Geometry: final body of the model. Coordinates: model frame, mm. A direction names the side the tool comes from. Give positions to 0.01 mm unless a question says otherwise; leave off trailing zeros. Write each loop counter-clockwise with the first axis right and the second up, starting at its lowest first coordinate (ties: lowest second). Pieces come first, ordered by that corner, then holes.
Q1. Section C-C (x = 12.5). Return the cut outline in (y, z).
Q2. Reachability of faces 4 (the cylindrical face through (-15.497, 3.441, 0.124)), 5 (the flat face through (5.474, -3.219, 3.881)), 6 (the flat face through (-10.304, 3.106, -7.638)), 7 (the cylindrical face through (-5.604, -14.23, -7.638)) from +Z, -Z, +X, -X, +Y, -Y: full face, straight path, thin tool, end or side. Return the list, or none.
Q3. Section B-B (y = -12). Return the cut outline in (x, z).
Q4. Mould query, pull axis Y, two halves, no side actions, for faces 1 (the cylindrical face through (-9.52, 11.97, -7.64)), 2 (the flat face through (7.88, -7.47, -7.64)), 3 (the flat face through (0, -13, -8.89)). Classes: +Y half, -Y half, draft (parallel to the pull), parting line (faces both ways), or undercut.
Q5. Section D-D (x = 5.5). Return the cut outline in (y, z).
Q6. Pin query (flat end, axial travel): pin 1 Ø5 at (y, z) = (4, -5.5) entering from +X; pin 2 Ø1.5 at (y, z) = (8, -5) entering from +X. Return the tip coordinate at first contact, or that it passes through.
Q7. Section A-A (z = 6). Return the cut outline in (x, y) (3 decimals).
Q8. Line query: line 1 (Y direction, x = 0, z = 2.25) (3 decimals); line 2 (X direction, y = 0, z = -0.75) (3 decimals); line 3 (Z direction, x = -4, y = -12). Output: solid intervals per line, ascending.
from build123d import *

# Parameters (mm, degrees)
BOSS_EXTRUDE1_DEPTH = 8.89
CUT_EXTRUDE1_DEPTH  = 10.16
CUT_EXTRUDE2_DEPTH  = 2.54


with BuildPart() as part:
    # Sketch1 → Boss-Extrude1 (new, symmetric)
    with BuildSketch(Plane.XY):
        with BuildLine():
            ThreePointArc((0, 15.875), (-15.875, 0), (0, -15.875))
            ThreePointArc((0, -15.875), (15.875, 0), (0, 15.875))
        make_face()
    extrude(amount=BOSS_EXTRUDE1_DEPTH, both=True)

    # Sketch2 → Cut-Extrude1 (cut)
    with BuildSketch(Plane.XY.offset(8.89)):
        Polygon((7.332348419, 0), (3.666174209, 6.35), (-3.666174209, 6.35), (-7.332348419, 0), (-3.666174209, -6.35), (3.666174209, -6.35), align=None)
    extrude(amount=-CUT_EXTRUDE1_DEPTH, mode=Mode.SUBTRACT)

    # Sketch4 → Cut-Extrude2 (cut)
    with BuildSketch(Plane(origin=(0, 0, -8.89), x_dir=(-1, 0, 0), z_dir=(0, 0, -1))):
        with BuildLine():
            Line((-6.379143124, 3.683), (-9.346003624, 11.161752295))
            ThreePointArc((-9.346003624, 11.161752295), (-8.255, 14.298079416), (-4.993359226, 13.674752709))
            Line((-4.993359226, 13.674752709), (0, 7.366))
            Line((0, 7.366), (4.993359226, 13.674752709))
            ThreePointArc((4.993359226, 13.674752709), (8.255, 14.298079416), (9.346003624, 11.161752295))
            Line((9.346003624, 11.161752295), (6.379143124, 3.683))
            Line((6.379143124, 3.683), (14.33936285, 2.513000415))
            ThreePointArc((14.33936285, 2.513000415), (16.51, 0), (14.33936285, -2.513000415))
            Line((14.33936285, -2.513000415), (6.379143124, -3.683))
            Line((6.379143124, -3.683), (9.346003624, -11.161752295))
            ThreePointArc((9.346003624, -11.161752295), (8.255, -14.298079416), (4.993359226, -13.674752709))
            Line((4.993359226, -13.674752709), (0, -7.366))
            Line((0, -7.366), (-4.993359226, -13.674752709))
            ThreePointArc((-4.993359226, -13.674752709), (-8.255, -14.298079416), (-9.346003624, -11.161752295))
            Line((-9.346003624, -11.161752295), (-6.379143124, -3.683))
            Line((-6.379143124, -3.683), (-14.33936285, -2.513000415))
            ThreePointArc((-14.33936285, -2.513000415), (-16.51, 0), (-14.33936285, 2.513000415))
            Line((-14.33936285, 2.513000415), (-6.379143124, 3.683))
        make_face()
    extrude(amount=-CUT_EXTRUDE2_DEPTH, mode=Mode.SUBTRACT)


solid = part.part
Computed:
1. outline: (-9.79, -8.89) - (-2.78, -8.89) - (-2.78, -6.35) - (2.78, -6.35) - (2.78, -8.89) - (9.79, -8.89) - (9.79, 8.89) - (-9.79, 8.89) - close
2. face 4: +Z, -Z
2. face 5: +Z
2. face 6: -Z
2. face 7: -Z, -X
3. outline: (-10.39, -8.89) - (-9.52, -8.89) - (-9.52, -6.35) - (-3.67, -6.35) - (-3.67, -8.89) - (3.67, -8.89) - (3.67, -6.35) - (9.52, -6.35) - (9.52, -8.89) - (10.39, -8.89) - (10.39, 8.89) - (-10.39, 8.89) - close
4. face 1: undercut
4. face 2: -Y half
4. face 3: draft
5. outline: (-14.89, -8.89) - (-14.16, -8.89) - (-14.16, -6.35) - (14.16, -6.35) - (14.16, -8.89) - (14.89, -8.89) - (14.89, 8.89) - (3.17, 8.89) - (3.17, -1.27) - (-3.17, -1.27) - (-3.17, 8.89) - (-14.89, 8.89) - close
6. pin 1: stops at x = 15.8
6. pin 2: stops at x = 14.12
7. outline: circle Ø31.75 at (0, 0); hole (-7.332, 0) - (-3.666, -6.35) - (3.666, -6.35) - (7.332, 0) - (3.666, 6.35) - (-3.666, 6.35) - close
8. line 1: y = -15.875 to -6.35, 6.35 to 15.875
8. line 2: x = -15.875 to -7.332, 7.332 to 15.875
8. line 3: z = -6.35 to 8.89
